The listing builds one solid part. Answer for the finished solid, in the listing's coordinates (mm). A direction names the side the tool comes from. Give positions to 0.01 mm unless a question says otherwise; leave off trailing zeros. Order: outer loops, then holes, each group sorted by start corner. A loop starts at its lowest first (then second) coordinate and runs counter-clockwise, first axis right, second up. Notation, with made-up numbers: (23, -5) - (64, -5) arc R23 cw to (64, 30) - close; hole circle Ø7 at (-26, -22). An arc over 180 degrees is marked (long way). Answer as CSV lines item,"result". Start each with the question number.
1. Determine the mould class of faces 1 (the flat face through (-19, -19, 1193.72)), 2 (the flat face through (-419.245, -19, 163)), 3 (the flat face through (-318, -35.56, -599)) for opening direction X: +X half, -X half, draft (parallel to the pull), parting line (faces both ways), or undercut.
2. Consider line 1 along X through (y, z) = (-4, 736); line 2 along Z through (x, y) = (115, -4). Determine where each line is inside the solid, lowest interval first. Write a range as [from, to].
3. Section B-B on z = 577 is taken. Give the vertices of the cut face in (x, y), and give its area (3 significant figures).
4. Which of the six approach directions +Z, -Z, +X, -X, +Y, -Y give full straight-line access (tool end or side, diameter ignored) to faces 4 (the flat face through (-317.645, -18, 206)), 5 (the flat face through (-68.3, -35.56, 1092.4))?
5. Section A-A on x = 33 is taken. Give the vertices of the cut face in (y, z).
6. Section C-C on y = -17.5 is taken. Count the separate pieces of the cut face and the enclosed holes in it, and give its area (3 significant figures).
from build123d import *

# Parameters (mm, degrees)
F0_W     = 812.8
F0_H     = 2032
F1_DEPTH = 38.1
F2_W     = 101.6
F2_H     = 101.6
F2_W_2   = 355.6
F2_H_2   = 1496.789953
F4_DEPTH = 309.88
F3_W     = 368.3
F3_H     = 1509.489953
F3_W_2   = 114.3
F3_H_2   = 114.3
F3_W_3   = 114.30002
F3_H_3   = 114.30002
F5_DEPTH = 2.54


with BuildPart() as f1:
    # F0 (on Front) → F1 (new body)
    with BuildSketch(Plane.XZ):
        with Locations((-12.845491, 177.719557)):
            Rectangle(F0_W, F0_H)
    extrude(amount=F1_DEPTH)

    # F2 (on face) → F4 (cut)
    with BuildSketch(Plane.XZ.offset(38.1)):
        with Locations((-266.845491, 1041.319557)):
            Rectangle(F2_W, F2_H)
        with Locations((-12.845491, 1041.319557)):
            Rectangle(F2_W_2, F2_H)
        with Locations((241.154509, 1041.319557)):
            Rectangle(F2_W, F2_H)
        with Locations((-266.845491, 216.724581)):
            Rectangle(F2_W, F2_H_2)
        with Locations((-12.845491, 216.724581)):
            Rectangle(F2_W_2, F2_H_2)
        with Locations((241.154509, 216.724581)):
            Rectangle(F2_W, F2_H_2)
        with Locations((-12.845491, -607.870396)):
            Rectangle(F2_W_2, F2_H)
        with Locations((241.154509, -607.870396)):
            Rectangle(F2_W, F2_H)
        with Locations((-266.845491, -607.870396)):
            Rectangle(F2_W, F2_H)
    extrude(amount=-F4_DEPTH, mode=Mode.SUBTRACT)

    # F3 (on face) → F5 (cut)
    with BuildSketch(Plane.XZ.offset(38.1)):
        with Locations((-12.845491, 216.724581)):
            Rectangle(F3_W, F3_H)
        with Locations((-266.845491, 216.724581)):
            Rectangle(F3_W_2, F3_H)
        with Locations((-266.845491, 1041.319557)):
            Rectangle(F3_W_2, F3_H_2)
        with Locations((-12.845491, 1041.319557)):
            Rectangle(F3_W, F3_H_2)
        with Locations((241.154509, 1041.319557)):
            Rectangle(F3_W_2, F3_H_2)
        with Locations((241.154509, 216.724581)):
            Rectangle(F3_W_2, F3_H)
        with Locations((241.154509, -607.870396)):
            Rectangle(F3_W_2, F3_H_2)
        with Locations((-12.845491, -607.870396)):
            Rectangle(F3_W, F3_H_2)
        with Locations((-266.845491, -607.870396)):
            Rectangle(F3_W_3, F3_H_3)
    extrude(amount=-F5_DEPTH, mode=Mode.SUBTRACT)


solid = f1.part
Checks:
1,face 1,"draft"
1,face 2,"-X half"
1,face 3,"undercut"
2,line 1,"x = [-419.25, -317.65], [-216.05, -190.65], [164.95, 190.35], [291.95, 393.55]"
2,line 2,"z = [-838.28, -658.67], [-557.07, -531.67], [965.12, 990.52], [1092.12, 1193.72]"
3,outline,"(-419.25, -38.1) - (-324, -38.1) - (-324, -35.56) - (-317.65, -35.56) - (-317.65, 0) - (-419.25, 0) - close; (-216.05, -35.56) - (-209.7, -35.56) - (-209.7, -38.1) - (-197, -38.1) - (-197, -35.56) - (-190.65, -35.56) - (-190.65, 0) - (-216.05, 0) - close; (164.95, -35.56) - (171.3, -35.56) - (171.3, -38.1) - (184, -38.1) - (184, -35.56) - (190.35, -35.56) - (190.35, 0) - (164.95, 0) - close; (291.95, -35.56) - (298.3, -35.56) - (298.3, -38.1) - (393.55, -38.1) - (393.55, 0) - (291.95, 0) - close"
3,area,"9,580 mm²"
4,face 4,"+Y, -Y"
4,face 5,"-Y"
5,outline,"(-38.1, -838.28) - (0, -838.28) - (0, -658.67) - (-35.56, -658.67) - (-35.56, -665.02) - (-38.1, -665.02) - close; (-38.1, -550.72) - (-35.56, -550.72) - (-35.56, -557.07) - (0, -557.07) - (0, -531.67) - (-35.56, -531.67) - (-35.56, -538.02) - (-38.1, -538.02) - close; (-38.1, 971.47) - (-35.56, 971.47) - (-35.56, 965.12) - (0, 965.12) - (0, 990.52) - (-35.56, 990.52) - (-35.56, 984.17) - (-38.1, 984.17) - close; (-38.1, 1098.47) - (-35.56, 1098.47) - (-35.56, 1092.12) - (0, 1092.12) - (0, 1193.72) - (-38.1, 1193.72) - close"
6,separate pieces,"1"
6,enclosed holes,"9"
6,area,"702,000 mm²"
